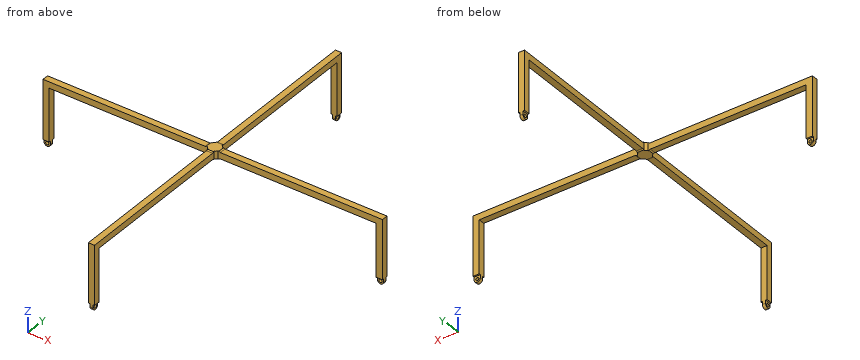
```python
from build123d import *

# Parameters (mm, degrees)
F0_R            = 5
F1_DEPTH        = 20
F2_T1_DEPTH     = 20
F4_COUNT        = 4
F3_R            = 20
F5_DEPTH        = 25
F6_R            = 5
F7_DEPTH        = 5
F7_COPIES_COUNT = 4
F8_W            = 20
F8_H            = 20
F9_DEPTH        = 5
F9_COPIES_COUNT = 4


# Not quite as in the source:
# - a fillet or chamfer that OpenCascade refuses, or shapes differently, is made with other operations: its cross-section is extruded or revolved along the edge and cut away or added
# - a pattern or mirror of a feature is missing from the dataset's text; its kind, count and spacing are read off the source's solid


with BuildPart() as f1:
    # F0 (on Front) → F1 (new body)
    with BuildSketch(Plane.XZ):
        with BuildLine():
            Line((0, 25), (0, 0))
            Line((0, 0), (20, 0))
            Line((20, 0), (20, 2.5))
            Line((20, 2.5), (525, 2.5))
            Line((525, 2.5), (525, -177.5))
            ThreePointArc((525, -177.5), (535, -187.5), (545, -177.5))
            Line((545, -177.5), (545, 22.5))
            Line((545, 22.5), (20, 22.5))
            Line((20, 22.5), (20, 25))
            Line((20, 25), (0, 25))
        make_face()
        with Locations((535, -177.5)):
            Circle(F0_R, mode=Mode.SUBTRACT)
    extrude(amount=F1_DEPTH)

    # F2: fillet of radius 5 on 2 edges, made by hand

    # F2_s2 → F2_t1 (join)
    with BuildSketch(Plane.XZ):
        with BuildLine():
            ThreePointArc((24.3301270189, 22.5), (21.8301270189, 23.1698729811), (20, 25))
            Line((20, 25), (20, 22.5))
            Line((20, 22.5), (24.3301270189, 22.5))
        make_face()
        with BuildLine():
            ThreePointArc((20, 0), (21.8301270189, 1.8301270189), (24.3301270189, 2.5))
            Line((24.3301270189, 2.5), (20, 2.5))
            Line((20, 2.5), (20, 0))
        make_face()
    extrude(amount=F2_T1_DEPTH)

    # F4: F1 ×4 about axis
    f4_axis = Axis((0, -10, 25), (0, 0, 1))


with BuildPart() as f1_1:
    add(f1.part)
    for i in range(1, F4_COUNT):
        add(f1.part.rotate(f4_axis, i * 360 / F4_COUNT))

    # F3 (on face) → F5 (join, through all)
    with BuildSketch(Plane.XY.offset(25)):
        with Locations((0, -10)):
            Circle(F3_R)
    extrude(amount=-F5_DEPTH)

    # F6 (on face) → F7 (cut)
    with BuildSketch(Plane(origin=(-10, 0, 0), x_dir=(0, -1, 0), z_dir=(-1, 0, 0))):
        with BuildLine():
            Line((555, -177.5), (555, -167.5))
            Line((555, -167.5), (535, -167.5))
            Line((535, -167.5), (535, -177.5))
            ThreePointArc((535, -177.5), (537.9289321881, -184.5710678119), (545, -187.5))
            ThreePointArc((545, -187.5), (552.0710678119, -184.5710678119), (555, -177.5))
        make_face()
        with Locations((545, -177.5)):
            Circle(F6_R, mode=Mode.SUBTRACT)
    f7 = extrude(amount=-F7_DEPTH, mode=Mode.SUBTRACT)

    # F7_copies: F7 ×4 about axis
    f7_copies_axis = Axis((0, -10, 0), (0, 0, 1))
    for i in range(1, F7_COPIES_COUNT):
        add(f7.rotate(f7_copies_axis, i * 360 / F7_COPIES_COUNT), mode=Mode.SUBTRACT)

    # F8 (on face) → F9 (cut)
    with BuildSketch(Plane.YZ.offset(10)):
        with Locations((-545, -177.5)):
            Rectangle(F8_W, F8_H)
    f9 = extrude(amount=-F9_DEPTH, mode=Mode.SUBTRACT)

    # F9_copies: F9 ×4 about axis
    f9_copies_axis = Axis((0, -10, 0), (0, 0, 1))
    for i in range(1, F9_COPIES_COUNT):
        add(f9.rotate(f9_copies_axis, i * 360 / F9_COPIES_COUNT), mode=Mode.SUBTRACT)


solid = f1_1.part
```
Input: part model. Units: mm. Frame: model coordinates. Coordinates: 2 decimals unless noted, no trailing zeros. Loops run counter-clockwise (first coordinate to the right, second up) from the corner with the lowest first, then second, coordinate; pieces in that order, holes last. Notation, with made-up numbers: M -26,44 L -20,44 A24 ccw -20,72 Z; hole C -31.5,18.5 d2. An arc over 180 degrees is marked long. Use a Markdown table: item, result. Add a question column.
1) Section A-A, the plane z = -18.5. Return the cut outline in (x, y), plus the area to 3 significant figures.
2) Section B-B, the plane x = -378.5. Return the cut outline in (y, z).
3) Line query: L1, parallel to Y at x = 1.25, z = -177.5; L2, parallel to Z at x = 2.25, y = 525; L3, parallel to Y at x = -7, z = -61. Output: solid intervals per line, ascending. Write a range as from..to.
4) Section C-C, the plane y = 234. Return the cut outline in (x, z).
5) Pin query (flat end, axial travel): P1, Ø1.5, axis at y = -50.5, z = 1, coming from the -X side; P2, Ø1.5, axis at x = 7.5, y = -547, coming from the -Z side; P3, Ø16, axis at y = -545, z = -177.5, coming from the -X side; P4, Ø16, axis at x = 229.5, y = -7.5, coming from the +Z side. Return the tip coordinate at first contact, or that it passes through.
Answer below:
| question | item | result |
|---|---|---|
| 1 | outline | M -545,-20 L -525,-20 L -525,0 L -545,0 Z; M -10,-555 L 10,-555 L 10,-535 L -10,-535 Z; M -10,515 L 10,515 L 10,535 L -10,535 Z; M 525,-20 L 545,-20 L 545,0 L 525,0 Z |
| 1 | area | 1,600 mm2 |
| 2 | outline | M -20,2.5 L 0,2.5 L 0,22.5 L -20,22.5 Z |
| 3 | L1 | -555..-550, -540..-535, 515..520, 530..535 |
| 3 | L2 | -187.5..-182.5, -172.5..22.5 |
| 3 | L3 | -555..-535, 515..535 |
| 4 | outline | M -10,2.5 L 10,2.5 L 10,22.5 L -10,22.5 Z |
| 5 | P1 | through |
| 5 | P2 | z = -167.5 |
| 5 | P3 | x = -5 |
| 5 | P4 | z = 22.5 |
